```python
from build123d import *

# Parameters (mm, degrees)
BASE_W              = 24.75
BASE_H              = 38
BASE_R              = 1.075
BOSS_EXTRUDE1_DEPTH = 5
SKETCH1_3_R         = 1.075
CUT_EXTRUDE1_DEPTH  = 2
SKETCH1_5_R         = 1.075
CUT_EXTRUDE2_DEPTH  = 24.219401909
FILLET1_R           = 2
CHAMFER1_SIZE       = 1
MOUNT_HOLE_R        = 1
CUT_EXTRUDE3_DEPTH  = 7.5


with BuildPart() as part:
    # Base → Boss-Extrude1 (new body)
    # profile 1 of 9: a face of its own
    with BuildSketch(Plane(origin=(0, 0, 0), x_dir=(1, 0, 0), z_dir=(0, 1, 0))):
        Rectangle(BASE_W, BASE_H)
        Polygon((-6.75, -12.809401077), (-4.75, -11.654700538), (-4.75, -9.345299462), (-6.75, -8.190598923), (-8.75, -9.345299462), (-8.75, -11.654700538), align=None, mode=Mode.SUBTRACT)
        Polygon((6.75, -12.809401077), (8.75, -11.654700538), (8.75, -9.345299462), (6.75, -8.190598923), (4.75, -9.345299462), (4.75, -11.654700538), align=None, mode=Mode.SUBTRACT)
        Polygon((8.75, 9.345299462), (8.75, 11.654700538), (6.75, 12.809401077), (4.75, 11.654700538), (4.75, 9.345299462), (6.75, 8.190598923), align=None, mode=Mode.SUBTRACT)
        Polygon((-6.75, 8.190598923), (-4.75, 9.345299462), (-4.75, 11.654700538), (-6.75, 12.809401077), (-8.75, 11.654700538), (-8.75, 9.345299462), align=None, mode=Mode.SUBTRACT)
    # profile 2 of 9: a face of its own
    with BuildSketch(Plane(origin=(0, 0, 0), x_dir=(1, 0, 0), z_dir=(0, 1, 0))):
        Polygon((4.75, -11.654700538), (6.75, -12.809401077), (8.75, -11.654700538), (8.75, -9.345299462), (6.75, -8.190598923), (4.75, -9.345299462), align=None)
        with Locations((6.75, -10.5)):
            Circle(BASE_R, mode=Mode.SUBTRACT)
    # profile 3 of 9: a face of its own
    with BuildSketch(Plane(origin=(0, 0, 0), x_dir=(1, 0, 0), z_dir=(0, 1, 0))):
        with Locations((6.75, -10.5)):
            Circle(BASE_R)
    # profile 4 of 9: a face of its own
    with BuildSketch(Plane(origin=(0, 0, 0), x_dir=(1, 0, 0), z_dir=(0, 1, 0))):
        Polygon((6.75, 8.190598923), (8.75, 9.345299462), (8.75, 11.654700538), (6.75, 12.809401077), (4.75, 11.654700538), (4.75, 9.345299462), align=None)
        with Locations((6.75, 10.5)):
            Circle(BASE_R, mode=Mode.SUBTRACT)
    # profile 5 of 9: a face of its own
    with BuildSketch(Plane(origin=(0, 0, 0), x_dir=(1, 0, 0), z_dir=(0, 1, 0))):
        Polygon((-8.75, 9.345299462), (-6.75, 8.190598923), (-4.75, 9.345299462), (-4.75, 11.654700538), (-6.75, 12.809401077), (-8.75, 11.654700538), align=None)
        with Locations((-6.75, 10.5)):
            Circle(BASE_R, mode=Mode.SUBTRACT)
    # profile 6 of 9: a face of its own
    with BuildSketch(Plane(origin=(0, 0, 0), x_dir=(1, 0, 0), z_dir=(0, 1, 0))):
        with Locations((-6.75, 10.5)):
            Circle(BASE_R)
    # profile 7 of 9: a face of its own
    with BuildSketch(Plane(origin=(0, 0, 0), x_dir=(1, 0, 0), z_dir=(0, 1, 0))):
        with Locations((6.75, 10.5)):
            Circle(BASE_R)
    # profile 8 of 9: a face of its own
    with BuildSketch(Plane(origin=(0, 0, 0), x_dir=(1, 0, 0), z_dir=(0, 1, 0))):
        Polygon((-8.75, -11.654700538), (-6.75, -12.809401077), (-4.75, -11.654700538), (-4.75, -9.345299462), (-6.75, -8.190598923), (-8.75, -9.345299462), align=None)
        with Locations((-6.75, -10.5)):
            Circle(BASE_R, mode=Mode.SUBTRACT)
    # profile 9 of 9: a face of its own
    with BuildSketch(Plane(origin=(0, 0, 0), x_dir=(1, 0, 0), z_dir=(0, 1, 0))):
        with Locations((-6.75, -10.5)):
            Circle(BASE_R)
    extrude(amount=BOSS_EXTRUDE1_DEPTH)

    # Sketch1<3> → Cut-Extrude1 (cut)
    # profile 1 of 8: a face of its own
    with BuildSketch(Plane(origin=(0, 0, 0), x_dir=(1, 0, 0), z_dir=(0, 1, 0))):
        Polygon((-8.75, 9.345299462), (-6.75, 8.190598923), (-4.75, 9.345299462), (-4.75, 11.654700538), (-6.75, 12.809401077), (-8.75, 11.654700538), align=None)
        with Locations((-6.75, 10.5)):
            Circle(SKETCH1_3_R, mode=Mode.SUBTRACT)
    # profile 2 of 8: a face of its own
    with BuildSketch(Plane(origin=(0, 0, 0), x_dir=(1, 0, 0), z_dir=(0, 1, 0))):
        with Locations((-6.75, 10.5)):
            Circle(SKETCH1_3_R)
    # profile 3 of 8: a face of its own
    with BuildSketch(Plane(origin=(0, 0, 0), x_dir=(1, 0, 0), z_dir=(0, 1, 0))):
        Polygon((-8.75, -11.654700538), (-6.75, -12.809401077), (-4.75, -11.654700538), (-4.75, -9.345299462), (-6.75, -8.190598923), (-8.75, -9.345299462), align=None)
        with Locations((-6.75, -10.5)):
            Circle(SKETCH1_3_R, mode=Mode.SUBTRACT)
    # profile 4 of 8: a face of its own
    with BuildSketch(Plane(origin=(0, 0, 0), x_dir=(1, 0, 0), z_dir=(0, 1, 0))):
        with Locations((-6.75, -10.5)):
            Circle(SKETCH1_3_R)
    # profile 5 of 8: a face of its own
    with BuildSketch(Plane(origin=(0, 0, 0), x_dir=(1, 0, 0), z_dir=(0, 1, 0))):
        Polygon((4.75, -11.654700538), (6.75, -12.809401077), (8.75, -11.654700538), (8.75, -9.345299462), (6.75, -8.190598923), (4.75, -9.345299462), align=None)
        with Locations((6.75, -10.5)):
            Circle(SKETCH1_3_R, mode=Mode.SUBTRACT)
    # profile 6 of 8: a face of its own
    with BuildSketch(Plane(origin=(0, 0, 0), x_dir=(1, 0, 0), z_dir=(0, 1, 0))):
        with Locations((6.75, -10.5)):
            Circle(SKETCH1_3_R)
    # profile 7 of 8: a face of its own
    with BuildSketch(Plane(origin=(0, 0, 0), x_dir=(1, 0, 0), z_dir=(0, 1, 0))):
        Polygon((6.75, 8.190598923), (8.75, 9.345299462), (8.75, 11.654700538), (6.75, 12.809401077), (4.75, 11.654700538), (4.75, 9.345299462), align=None)
        with Locations((6.75, 10.5)):
            Circle(SKETCH1_3_R, mode=Mode.SUBTRACT)
    # profile 8 of 8: a face of its own
    with BuildSketch(Plane(origin=(0, 0, 0), x_dir=(1, 0, 0), z_dir=(0, 1, 0))):
        with Locations((6.75, 10.5)):
            Circle(SKETCH1_3_R)
    extrude(amount=CUT_EXTRUDE1_DEPTH, mode=Mode.SUBTRACT)

    # Sketch1<5> → Cut-Extrude2 (cut, through all)
    with BuildSketch(Plane(origin=(0, 0, 0), x_dir=(1, 0, 0), z_dir=(0, 1, 0))):
        with Locations(Location((6.75, 10.5, 0), (0, 0, 270))):
            Circle(SKETCH1_5_R)
        with Locations(Location((6.75, -10.5, 0), (0, 0, 270))):
            Circle(SKETCH1_5_R)
        with Locations(Location((-6.75, -10.5, 0), (0, 0, 270))):
            Circle(SKETCH1_5_R)
        with Locations(Location((-6.75, 10.5, 0), (0, 0, 270))):
            Circle(SKETCH1_5_R)
    extrude(amount=CUT_EXTRUDE2_DEPTH, mode=Mode.SUBTRACT)

    # Fillet1
    fillet1_edges = [part.edges().sort_by_distance(p)[0] for p in [
        (12.375, 2.5, 19),
        (-12.375, 2.5, 19),
        (-12.375, 2.5, -19),
        (12.375, 2.5, -19),
    ]]
    fillet(fillet1_edges, radius=FILLET1_R)

    # Chamfer1
    # the kernel refuses this chamfer: 1 mm, written as the material it takes off along each edge
    with BuildSketch(Plane(origin=(12.375, 5, -19.571682988), x_dir=(0.027495876610585623, -0.9996219169112968, 0), z_dir=(0, 0, 1))) as chamfer1_piece_1:
        Polygon((CHAMFER1_SIZE * 0.999621916911, -CHAMFER1_SIZE * 0.0274958766106), (-CHAMFER1_SIZE * 0.0274958766106, -CHAMFER1_SIZE * 0.999621916911), (0, 0), align=None)
    extrude(amount=39.143365976, mode=Mode.SUBTRACT)
    with BuildSketch(Plane(origin=(-12.375, 5, 19.571682988), x_dir=(0.9996219169112968, 0.02749587661058651, 0), z_dir=(0, 0, -1))) as chamfer1_piece_2:
        Polygon((CHAMFER1_SIZE * 0.999621916911, CHAMFER1_SIZE * 0.0274958766106), (-CHAMFER1_SIZE * 0.0274958766106, CHAMFER1_SIZE * 0.999621916911), (0, 0), align=None)
    extrude(amount=39.143365976, mode=Mode.SUBTRACT)

    # Mount_Hole → Cut-Extrude3 (cut)
    with BuildSketch(Plane(origin=(0, 0, -19), x_dir=(-1, 0, 0), z_dir=(0, 0, -1))):
        with Locations((0, 2.5)):
            Circle(MOUNT_HOLE_R)
    cut_extrude3 = extrude(amount=-CUT_EXTRUDE3_DEPTH, mode=Mode.SUBTRACT)

    # Mirror1: Cut-Extrude3 across plane
    add(cut_extrude3.mirror(Plane(origin=(0, 0, 0), x_dir=(1, 0, 0), z_dir=(0, 0, -1))), mode=Mode.SUBTRACT)


solid = part.part
```
Model file for the job. Use its own axes, mm. A direction names the side the tool comes from. Give positions to 0.01 mm unless a question says otherwise; leave off trailing zeros. Loops run counter-clockwise (first coordinate to the right, second up) from the corner with the lowest first, then second, coordinate; pieces in that order, holes last. Notation, with made-up numbers: M -13.5,4.25 L 32.5,4.25 A30 cw 32.5,32.25 Z; hole C 11.25,-2.5 d11. An arc over 180 degrees is marked long. Use one line per item in the form item = value.
Item 1: Two-plate mould, pull along Y, no slides. Class faces 1 (the cylindrical face through (0.13, 3.49, 15.3)), 2 (the flat face through (8.75, 1, -10)), 3 (the flat face through (0, 5, 0)): released by +Y, released by -Y, zero draft, split by the parting line, or undercut.
Filled in:
face_1 = undercut
face_2 = zero draft
face_3 = released by +Y
Item 2: Slice it at C-C on x = 0. List the corners of the cut face in (y, z), and give its area (3 significant figures).
Filled in:
outline = M 0,-19 L 1.5,-19 L 1.5,-11.5 L 3.5,-11.5 L 3.5,-19 L 5,-19 L 5,19 L 3.5,19 L 3.5,11.5 L 1.5,11.5 L 1.5,19 L 0,19 Z
area = 160 mm^2
Item 3: Which spindle directions (+Z, -Z, +X, -X, +Y, -Y) get a long thin tool onto all of the face, cutting with end or side? Do faces 4 (the cylindrical face through (11.774, 2.535, 18.43)), 5 (the flat face through (5.76, 0.99, 8.76)), 6 (the flat face through (0, 3, -11.5)). Say none if no direction does.
Filled in:
face_4 = +Z, +X, +Y, -Y
face_5 = -Y
face_6 = -Z
Item 4: Slice it at A-A on z = 10.5. List the corners of the cut face in (x, y) (3 decimals).
Filled in:
outline = M -12.375,0 L -8.75,0 L -8.75,2 L -7.825,2 L -7.825,5 L -11.375,5 L -12.375,4 Z; M -5.675,2 L -4.75,2 L -4.75,0 L 4.75,0 L 4.75,2 L 5.675,2 L 5.675,5 L -5.675,5 Z; M 7.825,2 L 8.75,2 L 8.75,0 L 12.375,0 L 12.375,4 L 11.375,5 L 7.825,5 Z
Item 5: Slice it at B-B on x = 7.25. List the corners of the cut face in (y, z).
Filled in:
outline = M 0,-19 L 5,-19 L 5,-11.45 L 2,-11.45 L 2,-12.52 L 0,-12.52 Z; M 0,-8.48 L 2,-8.48 L 2,-9.55 L 5,-9.55 L 5,9.55 L 2,9.55 L 2,8.48 L 0,8.48 Z; M 0,12.52 L 2,12.52 L 2,11.45 L 5,11.45 L 5,19 L 0,19 Z
Item 6: Flat gauge pins, fed straight in: pin 1 Ø2 at (x, y) = (0, 2) entering from -Z; pin 2 Ø1.2 at (x, z) = (-7.5, -11) entering from -Y. Where does each tip first touch, or does it go through?
Filled in:
pin_1 = -19
pin_2 = 2
Item 7: Drill centre lines: L1, parallel to X at y = 3.3, z = 10.5 (3 decimals); L2, parallel to Z at x = 6.75, y = 2.7 (3 decimals); L3, parallel to Z at x = 7, y = 1.3. Where is each one in solid material? Low to high.
Filled in:
L1 = -12.375 to -7.825, -5.675 to 5.675, 7.825 to 12.375
L2 = -19 to -11.575, -9.425 to 9.425, 11.575 to 19
L3 = -19 to -12.67, -8.33 to 8.33, 12.67 to 19
